from build123d import *

# Parameters (mm, degrees)
SALIENTE_EXTRUIR1_DEPTH = 10
CROQUIS2_R              = 2
CORTAR_EXTRUIR1_DEPTH   = 213.132034356
CROQUIS3_W              = 70
CROQUIS3_H              = 8
SALIENTE_EXTRUIR2_DEPTH = 10


with BuildPart() as part:
    # Croquis1 → Saliente-Extruir1 (new body)
    with BuildSketch(Plane.XY):
        with BuildLine():
            Line((0, 0), (0, 200))
            Line((0, 200), (30, 200))
            ThreePointArc((30, 200), (37.071067812, 197.071067812), (40, 190))
            Line((40, 190), (40, 120))
            ThreePointArc((40, 120), (42.928932188, 112.928932188), (50, 110))
            Line((50, 110), (70, 110))
            Line((70, 110), (70, 0))
            Line((70, 0), (0, 0))
        make_face()
    extrude(amount=SALIENTE_EXTRUIR1_DEPTH)

    # Croquis2 → Cortar-Extruir1 (cut, through all)
    with BuildSketch(Plane.XY.offset(10)):
        with Locations((5, 195)):
            Circle(CROQUIS2_R)
        with Locations((5, 147.5)):
            Circle(CROQUIS2_R)
        with Locations((5, 100)):
            Circle(CROQUIS2_R)
        with Locations((5, 52.5)):
            Circle(CROQUIS2_R)
        with Locations((5, 5)):
            Circle(CROQUIS2_R)
        with Locations((64, 105)):
            Circle(CROQUIS2_R)
        with Locations((64, 55)):
            Circle(CROQUIS2_R)
        with Locations((64, 5)):
            Circle(CROQUIS2_R)
        with Locations((30, 195)):
            Circle(CROQUIS2_R)
        with Locations((30, 100)):
            Circle(CROQUIS2_R)
        with Locations((30, 5)):
            Circle(CROQUIS2_R)
    extrude(amount=-CORTAR_EXTRUIR1_DEPTH, mode=Mode.SUBTRACT)

    # Croquis3 → Saliente-Extruir2 (add)
    with BuildSketch(Plane.XY.offset(10)):
        with Locations((35, -4)):
            Rectangle(CROQUIS3_W, CROQUIS3_H)
    extrude(amount=-SALIENTE_EXTRUIR2_DEPTH)


solid = part.part
Source: CAD feature listing. Evaluate the final solid. Frame: model axes, mm. A direction names the side the tool comes from. Round coordinates to 2 decimals unless told otherwise and drop trailing zeros. Loops run counter-clockwise (first coordinate to the right, second up) from the corner with the lowest first, then second, coordinate; pieces in that order, holes last. Notation, with made-up numbers: (-31, 33.25) - (24, 33.25) arc R31 ccw to (24, 71.25) - close; hole circle Ø5 at (24.25, -33). An arc over 180 degrees is marked (long way). Write item = value, one per line. Start each with the question number.
(1) Section query A-A, the plane y = 147.5. Output: boundary loops of the cut face in (x, z).
(2) Section query D-D, the plane y = 195. Output: boundary loops of the cut face in (x, z), plus the area to 3 significant figures.
(3) Section query B-B, the plane x = 64. Output: boundary loops of the cut face in (y, z).
(4) Ray query, line 1 along Y through (x, z) = (30, 4.25); line 2 along Y through (x, z) = (64, 3.5); line 3 along Y through (x, z) = (60.5, 5). Return the intervals inside material, ascending. Write a range as from..to.
(5) Pin query (flat end, axial travel): pin 1 (5 mm diameter, centred on y = 141, z = 3, fed in from +X); pin 2 (5 mm diameter, centred on x = 64, y = 5, fed in from -Z). Return the tip coordinate at first contact, or that it passes through.
(6) Pull-direction query (Y, two-part tool) for faces 3 (the face through (42.85, 113.01, 4.93)), 4 (the face through (5, 102, 5)), 5 (the face through (27, 74, 10)); classes: +Y half, -Y half, draft (parallel to the pull), parting line (faces both ways), or undercut.
(7) Section query C-C, the plane z = 5. State how many separate pieces and enclosed holes the cut face has, plus the area to 3 significant figures.
(8) Set-up query: faces 1 (the face through (62, 5, 5)), 2 (the face through (60, 110, 5)). Return all of +Z, -Z, +X, -X, +Y, -Y with unobstructed straight access to the full face (end or side cutting, diameter ignored); none if empty.
Conclusion:
q1.outline = (0, 0) - (3, 0) - (3, 10) - (0, 10) - close; (7, 0) - (40, 0) - (40, 10) - (7, 10) - close
q2.outline = (0, 0) - (3, 0) - (3, 10) - (0, 10) - close; (7, 0) - (28, 0) - (28, 10) - (7, 10) - close; (32, 0) - (38.66, 0) - (38.66, 10) - (32, 10) - close
q2.area = 307 mm2
q3.outline = (-8, 0) - (3, 0) - (3, 10) - (-8, 10) - close; (7, 0) - (53, 0) - (53, 10) - (7, 10) - close; (57, 0) - (103, 0) - (103, 10) - (57, 10) - close; (107, 0) - (110, 0) - (110, 10) - (107, 10) - close
q4.line_1 = -8..3, 7..98, 102..193, 197..200
q4.line_2 = -8..3, 7..53, 57..103, 107..110
q4.line_3 = -8..110
q5.pin_1 = 40
q5.pin_2 = 0
q6.face_3 = +Y half
q6.face_4 = undercut
q6.face_5 = draft
q7.separate_pieces = 1
q7.enclosed_holes = 11
q7.area = 11,700 mm2
q8.face_1 = +Z, -Z
q8.face_2 = +Z, -Z, +X, +Y
